Read the model definition and answer for the solid it produces. Units are mm, in the model's axes. A direction names the side the tool comes from. Round coordinates to 2 decimals unless told otherwise and drop trailing zeros. Order: outer loops, then holes, each group sorted by start corner. A loop starts at its lowest first (then second) coordinate and runs counter-clockwise, first axis right, second up. Notation, with made-up numbers: (-32.5, -40) - (4.5, -40) arc R15 ccw to (4.5, -34) - close; hole circle Ø6 at (-5, 25.25). An arc over 180 degrees is marked (long way). Answer as a JSON object with one key per item and string values. Group by question number.
Q1. The mould has two halves that part along Z. Classify faces 3 (the cylindrical face through (6.237, 8.584, 0.696)), 4 (the cylindrical face through (8.09, 11.46, 0.2)), 5 (the flat face through (9, 11, 0.4)), 6 (the flat face through (10, 9, 0)): pulls with the +Z half, pulls with the -Z half, needs draft (parallel to the pull), parting line crosses it, or undercut.
Q2. A tool of negligible diameter and unlimited length cuts with its end or side. For faces 1 (the flat face through (9, 11, 1)), 2 (the cylindrical face through (8.09, 11.46, 1.2)), from which of +Z, -Z, +X, -X, +Y, -Y can it reach the whole face along a straight path? Write none if from no direction.
Q3. Consider line 1 (X direction, y = 8.55, z = 0.6); line 2 (Y direction, x = 8.5, z = 0.3); line 3 (Z direction, x = 6, y = 7.75). Determine where each line is inside the solid, lowest interval first.
Q4. A cutting plane is placed at C-C on x = 9.8. Determine the outline of the cut face in (y, z).
Q5. A cutting plane is placed at B-B on x = 8.1. Determine the outline of the cut face in (y, z), and give its area (3 significant figures).
Q6. A cutting plane is placed at A-A on y = 9.55. Determine the outline of the cut face in (x, z), and give its area (3 significant figures).
Q7. A cutting plane is placed at D-D on y = 6.4. Determine the outline of the cut face in (x, z).
```python
from build123d import *

# Parameters (mm, degrees)
SKETCH1_R           = 3
SKETCH1_R_2         = 2.25
SKETCH1_R_3         = 1.2
BOSS_EXTRUDE1_DEPTH = 0.4
BOSS_EXTRUDE4_START = 0.4
SKETCH1_8_R         = 2.25
SKETCH1_8_R_2       = 1.2
BOSS_EXTRUDE4_DEPTH = 0.6
BOSS_EXTRUDE5_START = 1
SKETCH1_9_R         = 3
SKETCH1_9_R_2       = 2.25
SKETCH1_9_R_3       = 1.2
BOSS_EXTRUDE5_DEPTH = 0.4


with BuildPart() as part:
    # Sketch1 → Boss-Extrude1 (new body)
    # profile 1 of 2: a face of its own
    with BuildSketch(Plane.XY):
        with Locations((8.485, 8.485)):
            Circle(SKETCH1_R)
        with Locations((8.485, 8.485)):
            Circle(SKETCH1_R_2, mode=Mode.SUBTRACT)
    # profile 2 of 2: a face of its own
    with BuildSketch(Plane.XY):
        with Locations((8.485, 8.485)):
            Circle(SKETCH1_R_2)
        with Locations((8.485, 8.485)):
            Circle(SKETCH1_R_3, mode=Mode.SUBTRACT)
    extrude(amount=BOSS_EXTRUDE1_DEPTH)

    # Sketch1<8> → Boss-Extrude4 (add)
    with BuildSketch(Plane.XY.offset(BOSS_EXTRUDE4_START)):
        with Locations((8.485, 8.485)):
            Circle(SKETCH1_8_R)
        with Locations((8.485, 8.485)):
            Circle(SKETCH1_8_R_2, mode=Mode.SUBTRACT)
    extrude(amount=BOSS_EXTRUDE4_DEPTH)

    # Sketch1<9> → Boss-Extrude5 (add)
    # profile 1 of 2: a face of its own
    with BuildSketch(Plane.XY.offset(BOSS_EXTRUDE5_START)):
        with Locations((8.485, 8.485)):
            Circle(SKETCH1_9_R)
        with Locations((8.485, 8.485)):
            Circle(SKETCH1_9_R_2, mode=Mode.SUBTRACT)
    # profile 2 of 2: a face of its own
    with BuildSketch(Plane.XY.offset(BOSS_EXTRUDE5_START)):
        with Locations((8.485, 8.485)):
            Circle(SKETCH1_9_R_2)
        with Locations((8.485, 8.485)):
            Circle(SKETCH1_9_R_3, mode=Mode.SUBTRACT)
    extrude(amount=BOSS_EXTRUDE5_DEPTH)


solid = part.part
```
Result set:
{
 "1": {"face 3": "undercut", "face 4": "needs draft", "face 5": "undercut", "face 6": "pulls with the -Z half"},
 "2": {"face 1": "none", "face 2": "+Z, -Z"},
 "3": {"line 1": "x = 6.24 to 7.29, 9.68 to 10.73", "line 2": "y = 5.49 to 7.29, 9.68 to 11.48", "line 3": "z = 0 to 0.4, 1 to 1.4"},
 "4": {"outline": "(5.79, 0) - (11.18, 0) - (11.18, 0.4) - (10.31, 0.4) - (10.31, 1) - (11.18, 1) - (11.18, 1.4) - (5.79, 1.4) - (5.79, 1) - (6.66, 1) - (6.66, 0.4) - (5.79, 0.4) - close"},
 "5": {"outline": "(5.51, 0) - (7.35, 0) - (7.35, 1.4) - (5.51, 1.4) - (5.51, 1) - (6.27, 1) - (6.27, 0.4) - (5.51, 0.4) - close; (9.62, 0) - (11.46, 0) - (11.46, 0.4) - (10.7, 0.4) - (10.7, 1) - (11.46, 1) - (11.46, 1.4) - (9.62, 1.4) - close", "area": "4.24 mm²"},
 "6": {"outline": "(5.68, 0) - (7.93, 0) - (7.93, 1.4) - (5.68, 1.4) - (5.68, 1) - (6.5, 1) - (6.5, 0.4) - (5.68, 0.4) - close; (9.04, 0) - (11.29, 0) - (11.29, 0.4) - (10.47, 0.4) - (10.47, 1) - (11.29, 1) - (11.29, 1.4) - (9.04, 1.4) - close", "area": "5.32 mm²"},
 "7": {"outline": "(6.33, 0) - (10.64, 0) - (10.64, 0.4) - (9.33, 0.4) - (9.33, 1) - (10.64, 1) - (10.64, 1.4) - (6.33, 1.4) - (6.33, 1) - (7.64, 1) - (7.64, 0.4) - (6.33, 0.4) - close"}
}
